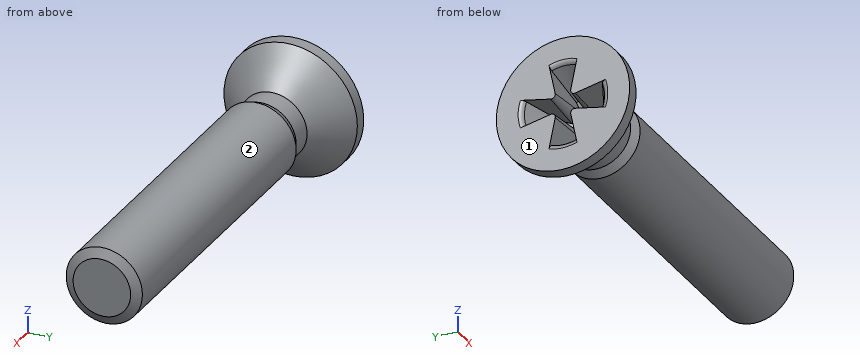
Autodesk Inventor part; units mm, degrees
ref_plane "Work Plane2" through (3.35, 0, 0) normal (0, 0, -1) x (1, 0, 0)
ref_plane "YZ Plane" through (0, 0, 0) normal (1, 0, 0) x (0, 1, 0)
ref_plane "XZ Plane" through (0, 0, 0) normal (0, 1, 0) x (-1, 0, 0)
sketch "Sketch1" plane through (0, 0, 0) normal (0, 0, 1) x (1, 0, 0)
  line L0 (1.32, 0) -> (10, 0)
  line L1 (10, 0) -> (10, 1)
  line L2 (10, 1) -> (2, 1)
  line L3 (2, 1) -> (1.7546, 0.8773)
  line L4 (1.7546, 0.8773) -> (1.2, 0.8773)
  line L5 (0, 1.75) -> (0, 1.09)
  line L6 (0, 1.09) -> (1.0075, 0.5877)
  line L7 (1.0075, 0.5877) -> (1.32, 0)
  line L8 (-2, 0) -> (12, 0)
  line L9 (0, -0.35) -> (0, 2.1)
  line L10 (0, 1.75) -> (0.3273, 1.75)
  line L11 (0.3273, 1.75) -> (1.2, 0.8773)
  line L12 (2, 1) -> (1.0773, 1) construction
  dimension "d1" = 8
  dimension "d2" = 2
  dimension "d3" = 1.7546
  dimension "d4" = 2.18
  dimension "d5" = 26.5
  dimension "d6" = 62
  dimension "d7" = 1.32
  dimension "d8" = 0.2454
  dimension "d12" = 3.5
  dimension "d13" = 45
  dimension "d15" = 10
  dimension "d24" = 1.2
revolve "Body" add sketch "Sketch1" angle 360 about axis through (1.32, 0, 0) along (1, 0, 0) contours L7 L6 L5 L10 L11 L4 L3 L2 L1 L0
sketch "Sketch2" plane through (0, 0, 0) normal (-1, 0, 0) x (0, 0, 1)
  line L0 (0, 1.09) -> (0, 0) construction
  line L1 (0, 0) -> (1.09, 0) construction
  arc A0 (0.327, 0) -> (0, 0.327) centre (0, 0) ccw construction
  arc A1 (0.3815, 0) -> (0, 0.3815) centre (0, 0) ccw construction
  arc A2 (1.0323, 0.35) -> (0.35, 1.0323) centre (0, 0) ccw
  line L2 (0, 0) -> (0.7707, 0.7707) construction
  line L3 (0.35, 1.0323) -> (0.2039, 0.3225)
  line L4 (1.0323, 0.35) -> (0.3225, 0.2039)
  arc A3 (0.35, 1.0323) -> (0, 1.09) centre (0, 0) ccw
  arc A4 (1.09, 0) -> (1.0323, 0.35) centre (0, 0) ccw
  line L5 (0, -2.45) -> (0, 2.45)
  line L6 (-2.45, 0) -> (2.45, 0)
  arc A5 (0.35, -1.0323) -> (1.0323, -0.35) centre (0, 0) ccw
  line L7 (0.35, -1.0323) -> (0.2039, -0.3225)
  line L8 (1.0323, -0.35) -> (0.3225, -0.2039)
  arc A6 (0, -1.09) -> (0.35, -1.0323) centre (0, 0) ccw
  arc A7 (1.0323, -0.35) -> (1.09, 0) centre (0, 0) ccw
  arc A8 (-0.35, 1.0323) -> (-1.0323, 0.35) centre (0, 0) ccw
  line L9 (-0.35, 1.0323) -> (-0.2039, 0.3225)
  line L10 (-1.0323, 0.35) -> (-0.3225, 0.2039)
  arc A9 (0, 1.09) -> (-0.35, 1.0323) centre (0, 0) ccw
  arc A10 (-1.0323, 0.35) -> (-1.09, 0) centre (0, 0) ccw
  arc A11 (-0.35, -1.0323) -> (0, -1.09) centre (0, 0) ccw
  arc A12 (-1.0323, -0.35) -> (-0.35, -1.0323) centre (0, 0) ccw
  arc A13 (-1.09, 0) -> (-1.0323, -0.35) centre (0, 0) ccw
  line L11 (-1.0323, -0.35) -> (-0.3225, -0.2039)
  line L12 (-0.35, -1.0323) -> (-0.2039, -0.3225)
  arc A14 (0.2039, 0.3225) -> (0.3225, 0.2039) centre (0.3022, 0.3022) ccw
  arc A15 (0.3225, -0.2039) -> (0.2039, -0.3225) centre (0.3022, -0.3022) ccw
  arc A16 (-0.3225, 0.2039) -> (-0.2039, 0.3225) centre (-0.3022, 0.3022) ccw
  arc A17 (-0.2039, -0.3225) -> (-0.3225, -0.2039) centre (-0.3022, -0.3022) ccw
  point P0 (0.7707, -0.7707)
  point P1 (-0.7707, 0.7707)
  point P2 (-0.7707, -0.7707)
  dimension "d17" = 0.654
  dimension "d18" = 0.763
  dimension "d19" = 2.18
  dimension "d20" = 45
  dimension "d21" = 0.35
extrude "Slot" add sketch "Sketch2" against normal up to next draft 5 contours L4 A14 L3 A2 | A5 L7 A15 L8 | L9 A16 L10 A8 | A12 L11 A17 L12
fillet "Fillet1" radius 0.14 4 edges at (0, 1.09, 0) (0, 0, -1.09) (0, -1.09, 0) (0, 0, 1.09)
thread "Thread"
chamfer "Chamfer1" distance 0.2454 distance2 0.1227 1 edges at (10, -1, 0) measured on face at (10, -0.0858, 0.7069)
ref_plane "Work Plane2" through (3.35, 0, 0) normal (0, 0, -1) x (1, 0, 0)
equation "\"d17\" = 0.3 * SDM"
equation "\"d18\" = 0.35 * SDM"
equation "\"d19\" = SDM"
equation "\"d21\" = 0.5 * SBR"
equation "\"d1\" = GEL"
equation "\"d2\" = GD"
equation "\"d3\" = BDM"
equation "\"d4\" = SDM"
equation "\"d7\" = INTI"
equation "\"d8\" = GAL"
equation "\"d12\" = KOD"
equation "\"d13\" = 0.5 * SEWI"
equation "\"d15\" = NLG"
equation "\"d24\" = KOH"
equation "\"d23\" = 0.2 * SBR"
equation "\"d10\" = GEL"
equation "\"d25\" = -0.5 * SPD + 0.5 * GD"
equation "\"d26\" = 0.5 * GAL"
equation "\"NLG\" = 10"
equation "\"GEL\" = 8"
equation "\"GAL\" = 0.61345 * PTC"
equation "\"SPD\" = NND - 1.2269 * PTC"
equation "\"KOD\" = 3.5"
equation "\"KOH\" = 1.2"
equation "\"SBR\" = 0.7"
equation "\"INTI\" = 1.32"
equation "\"SDM\" = 2.18"
equation "\"GD\" = NND"
equation "\"BDM\" = NND - GAL"
equation "\"SEWI\" = 90deg"
equation "\"d9\" = SDM"
equation "\"GUL\" = 0.61345 * PTC"
equation "\"TOA\" = 30deg"
equation "\"EPV\" = 2.2"
equation "\"THREADDIA\" = 2"
equation "\"RR\" = 0.2"
equation "\"PTC\" = 0.4"
equation "\"NND\" = 2"
equation "\"GD1\" = THREADDIA - 1.2269 * PTC"
properties part number "AS 1427 - M2 x 10" material "Steel, Mild"
Read the model definition and answer for the solid it produces. Units are mm, in the model's axes. Face numbers are marked on the shaded views. A direction names the side the tool comes from. Give positions to 0.01 mm unless a question says otherwise; leave off trailing zeros. Order: outer loops, then holes, each group sorted by start corner. A loop starts at its lowest first (then second) coordinate and runs counter-clockwise, first axis right, second up.
(1) Straight lines are drawn through the part: L1, parallel to Z at x = 3.25, y = -0.05; L2, parallel to Z at x = 3.5, y = 0.7; L3, parallel to X at y = 0.55, z = -1.4. For each, find the intervals that lie inside material, in ascending order.
(2) Find section B-B (x = 8.5). Give the vertices of the cut face in (y, z), plus the area to 3 significant figures.
(3) For the marked faces 1 and 2, determine the directions among +Z, -Z, +X, -X, +Y, -Y from which every point of the face is accessible in a straight line to the end or side of a thin tool.
(4) Find section A-A (x = 0.5). Give the vertices of the cut face in (y, z), plus the area to 3 significant figures.
(5) Given pin 1 (1.5 mm diameter, centred on x = 6.5, y = -0.5, fed in from -Z); pin 2 (1.5 mm diameter, centred on x = 6.5, z = 0, fed in from -Y); pin 3 (2 mm diameter, centred on x = 1.5, z = -0.5, fed in from -Y), each flat-ended and moving along its own axis, determine where each tip first touches the part or whether it passes through.
Result sheet:
1. L1: z = -1 to 1
1. L2: z = -0.71 to 0.71
1. L3: x = 0 to 0.57
2. outline: circle Ø2 at (0, 0)
2. area: 3.14 mm2
3. face 1: +Z, -Z, -X, +Y, -Y
3. face 2: +X
4. outline: circle Ø3.15 at (0, 0); hole (-0.8, -0.26) - (-0.33, -0.16) arc R0.14 cw to (-0.16, -0.33) - (-0.26, -0.8) arc R0.84 ccw to (0.26, -0.8) - (0.16, -0.33) arc R0.14 cw to (0.33, -0.16) - (0.8, -0.26) arc R0.84 ccw to (0.8, 0.26) - (0.33, 0.16) arc R0.14 cw to (0.16, 0.33) - (0.26, 0.8) arc R0.84 ccw to (-0.26, 0.8) - (-0.16, 0.33) arc R0.14 cw to (-0.33, 0.16) - (-0.8, 0.26) arc R0.84 ccw to start
4. area: 6.64 mm2
5. pin 1: stops at z = -1
5. pin 2: stops at y = -1
5. pin 3: stops at y = -1.53
